Design review of the part built by this model. Coordinates are the model's own, in mm. Face numbers are marked on the shaded views. Coordinates: 2 decimals unless noted, no trailing zeros. Loops run counter-clockwise (first coordinate to the right, second up) from the corner with the lowest first, then second, coordinate; pieces in that order, holes last.
Q1. Add section B-B on z = 0. Give the boundary of the cut face in (x, y), and give its area (3 significant figures).
Q2. Draft analysis for pull direction Z (two halves, no side actions). For the marked faces 1, 2 and 3, state which applies: released by +Z, released by -Z, zero draft, split by the parting line, or undercut.
Q3. Add section C-C on z = 4.5. Give the boundary of the cut face in (x, y), and give its area (3 significant figures).
Q4. Wall thickness on probe 1 along X at (y, z) = (-5, 3.75); probe 2 along X at (y, z) = (-1.25, 4.75); probe 3 along Z at (x, y) = (-6, -2.5): over which ranges is each line inside the solid? List them lowest first.
Q5. For P1, Ø2, axis at y = -5.5, z = 2.5, coming from the +X side; P2, Ø3, axis at x = -3, y = -4.5, coming from the -Z side; P3, Ø1.5, axis at x = 5.5, y = -3.5, coming from the +Z side, all flat-tipped, find the tip position at first contact; note any pin that passes through.
```python
from build123d import *

# Parameters (mm, degrees)
F0_R     = 2.54
F1_DEPTH = 6.35


with BuildPart() as f1:
    # F0 (on Front) → F1 (new body)
    with BuildSketch(Plane.XZ):
        with BuildLine():
            ThreePointArc((-4.468796, 8.440379), (-5.206836, 6.566125), (-7.199962, 6.274607))
            ThreePointArc((-7.199962, 6.274607), (-7.356389, 6.090459), (-7.508107, 5.902412))
            ThreePointArc((-7.508107, 5.902412), (-7.422522, 3.889899), (-9.126103, 2.81503))
            ThreePointArc((-9.126103, 2.81503), (-9.194395, 2.583262), (-9.256802, 2.349841))
            ThreePointArc((-9.256802, 2.349841), (-8.362303, 0.545014), (-9.483499, -1.128441))
            ThreePointArc((-9.483499, -1.128441), (-9.451918, -1.367987), (-9.414286, -1.606659))
            ThreePointArc((-9.414286, -1.606659), (-7.864634, -2.893558), (-8.210717, -4.877936))
            ThreePointArc((-8.210717, -4.877936), (-8.08469, -5.084085), (-7.953489, -5.28698))
            ThreePointArc((-7.953489, -5.28698), (-6.015063, -5.834737), (-5.526542, -7.788933))
            ThreePointArc((-5.526542, -7.788933), (-5.327734, -7.926247), (-5.125515, -8.058488))
            ThreePointArc((-5.125515, -8.058488), (-3.131525, -7.772946), (-1.892375, -9.361039))
            ThreePointArc((-1.892375, -9.361039), (-1.654959, -9.405916), (-1.416485, -9.444772))
            ThreePointArc((-1.416485, -9.444772), (0.290311, -8.375014), (2.067085, -9.324017))
            ThreePointArc((2.067085, -9.324017), (2.302297, -9.268742), (2.536035, -9.207533))
            ThreePointArc((2.536035, -9.207533), (3.662244, -7.537447), (5.67122, -7.684231))
            ThreePointArc((5.67122, -7.684231), (5.863796, -7.538304), (6.052619, -7.387553))
            ThreePointArc((6.052619, -7.387553), (6.40465, -5.404221), (8.300493, -4.723552))
            ThreePointArc((8.300493, -4.723552), (8.417331, -4.51206), (8.52878, -4.297679))
            ThreePointArc((8.52878, -4.297679), (8.04612, -2.342028), (9.502942, -0.950913))
            ThreePointArc((9.502942, -0.950913), (9.523956, -0.710209), (9.538875, -0.46905))
            ThreePointArc((9.538875, -0.46905), (8.304491, 1.122751), (9.071869, 2.985185))
            ThreePointArc((9.071869, 2.985185), (8.993448, 3.213725), (8.909271, 3.440207))
            ThreePointArc((8.909271, 3.440207), (7.13535, 4.394533), (7.081375, 6.408141))
            ThreePointArc((7.081375, 6.408141), (6.916999, 6.585231), (6.748196, 6.758105))
            ThreePointArc((6.748196, 6.758105), (4.739669, 6.91091), (3.873618, 8.72956))
            ThreePointArc((3.873618, 8.72956), (3.651543, 8.824759), (3.427131, 8.91431))
            ThreePointArc((3.427131, 8.91431), (1.529255, 8.239328), (0, 9.5504))
            ThreePointArc((0, 9.5504), (-0.330856, 9.544667), (-0.661315, 9.527476))
            ThreePointArc((-0.661315, 9.527476), (-2.096114, 8.113658), (-4.036173, 8.655602))
            ThreePointArc((-4.036173, 8.655602), (-4.253846, 8.550727), (-4.468796, 8.440379))
        make_face()
        Circle(F0_R, mode=Mode.SUBTRACT)
    extrude(amount=F1_DEPTH)


solid = f1.part
```
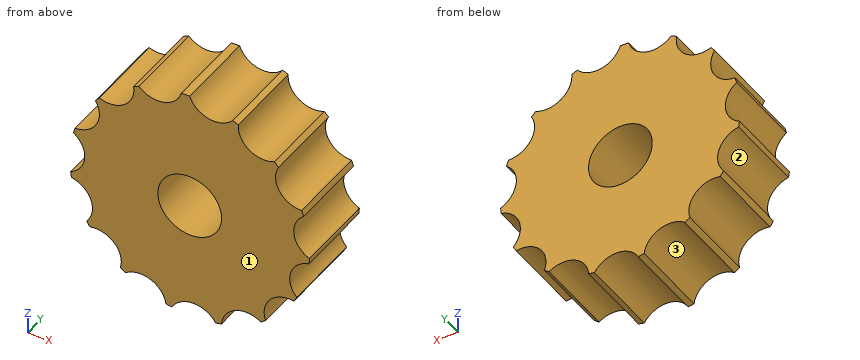
Entries:
1. outline: (-8.48, -6.35) - (-2.54, -6.35) - (-2.54, 0) - (-8.48, 0) - close; (2.54, -6.35) - (8.85, -6.35) - (8.85, 0) - (2.54, 0) - close
1. area: 77.7 mm2
2. face 1: zero draft
2. face 2: undercut
2. face 3: released by -Z
3. outline: (-7.22, -6.35) - (7.07, -6.35) - (7.07, 0) - (-7.22, 0) - close
3. area: 90.8 mm2
4. probe 1: x = -7.5 to 7.77
4. probe 2: x = -7.19 to 6.96
4. probe 3: z = -5.85 to 6.18
5. P1: stops at x = 9.07
5. P2: stops at z = -9.43
5. P3: stops at z = 6.9
